```python
from build123d import *

# Parameters (mm, degrees)
SKETCH2_W               = 30
SKETCH2_H               = 18.5
BOSS_EXTRUDE1_DEPTH     = 4.5
BOSS_EXTRUDE2_DEPTH     = 5
SKETCH4_W               = 26.3
SKETCH4_H               = 37.3
BOSS_EXTRUDE3_DEPTH     = 9
SKETCH5_W               = 30
SKETCH5_H               = 40.415903306
SKETCH5_W_2             = 26.3
SKETCH5_H_2             = 37.3
BOSS_EXTRUDE4_DEPTH     = 2
CUT_EXTRUDE1_DEPTH      = 53.877515324
SKETCH7_R               = 2.75
CUT_EXTRUDE2_DEPTH      = 3
SKETCH8_R               = 1.65
CUT_EXTRUDE3_DEPTH      = 51.656012741
SKETCH9_W               = 0.2
SKETCH9_H               = 4
TOLERANCE_CUT1_DEPTH    = 53.877515324
TOLERANCE_CUT2_DEPTH    = 0.2
SKETCH12_W              = 26.022193388
SKETCH12_H              = 26.438096694
BOSS_EXTRUDE6_DEPTH     = 1.5
SKETCH13_W              = 28.011096694
SKETCH13_H              = 28.427
BOSS_EXTRUDE7_DEPTH     = 1.5
SKETCH16_W              = 1.5
SKETCH16_H              = 1.5
SILICONE_CHANNELS_DEPTH = 3
SKETCH19_W              = 19.3
SKETCH19_H              = 15.3
PCB_CAVITY_DEPTH        = 1.7
SKETCH15_R              = 1
PCB_MOUNT_HOLES_DEPTH   = 5
SKETCH20_W              = 5
SKETCH20_H              = 15.3
SOLDER_CAVITY_DEPTH     = 1.2
SKETCH21_R              = 0.5
AUDIO_CHANNEL_DEPTH     = 50.204386256
SKETCH22_R              = 3.5
CUT_EXTRUDE13_DEPTH     = 52.193570171


with BuildPart() as part:
    # Sketch2 → Boss-Extrude1 (new body)
    with BuildSketch(Plane.XY):
        with Locations((13, -1.25)):
            Rectangle(SKETCH2_W, SKETCH2_H)
    extrude(amount=BOSS_EXTRUDE1_DEPTH)

    # Sketch3 → Boss-Extrude2 (add)
    with BuildSketch(Plane.XY.offset(4.5)):
        Polygon((-2, 38.415903306), (28, 38.415903306), (28, -6), (22.890598923, -6), (25.2, -2), (0.7, -2), (3.009401077, -6), (-2, -6), align=None)
    extrude(amount=BOSS_EXTRUDE2_DEPTH)

    # Sketch4 → Boss-Extrude3 (add)
    with BuildSketch(Plane.XY.offset(9.5)):
        Polygon((-2, 38.415903306), (-2, -6), (3.009401077, -6), (0.7, -2), (25.2, -2), (22.890598923, -6), (28, -6), (28, 38.415903306), align=None)
        with Locations((13, 18.5)):
            Rectangle(SKETCH4_W, SKETCH4_H, mode=Mode.SUBTRACT)
    extrude(amount=BOSS_EXTRUDE3_DEPTH)

    # Sketch5 → Boss-Extrude4 (add)
    with BuildSketch(Plane.XY.offset(18.5)):
        with Locations((13, 18.207951653)):
            Rectangle(SKETCH5_W, SKETCH5_H)
        with Locations((13, 18.5)):
            Rectangle(SKETCH5_W_2, SKETCH5_H_2, mode=Mode.SUBTRACT)
    extrude(amount=BOSS_EXTRUDE4_DEPTH)

    # Sketch6 → Cut-Extrude1 (cut, through all)
    with BuildSketch(Plane(origin=(28, 0, 0), x_dir=(0, 0, -1), z_dir=(1, 0, 0))):
        with BuildLine():
            Line((-12.5, 38.415903306), (-29.920257518, 38.415903306))
            Line((-29.920257518, 38.415903306), (-29.920257518, -0.15))
            Line((-29.920257518, -0.15), (-20.5, -0.15))
            ThreePointArc((-20.5, -0.15), (-19.694107493, 6.728151663), (-17.320084205, 13.23372208))
            ThreePointArc((-17.320084205, 13.23372208), (-13.721563712, 23.094799932), (-12.5, 33.520632668))
            Line((-12.5, 33.520632668), (-12.5, 38.415903306))
        make_face()
    extrude(amount=-CUT_EXTRUDE1_DEPTH, mode=Mode.SUBTRACT)

    # Sketch7 → Cut-Extrude2 (cut)
    with BuildSketch(Plane(origin=(0, 0, 0), x_dir=(-1, 0, 0), z_dir=(0, 0, -1))):
        with Locations((-19.5, -6.25)):
            Circle(SKETCH7_R)
        with Locations(Location((-6.5, -6.25, 0), (0, 0, 180))):
            Circle(SKETCH7_R)
    extrude(amount=-CUT_EXTRUDE2_DEPTH, mode=Mode.SUBTRACT)

    # Sketch8 → Cut-Extrude3 (cut, through all)
    with BuildSketch(Plane(origin=(0, 0, 3), x_dir=(-1, 0, 0), z_dir=(0, 0, -1))):
        with Locations((-19.5, -6.25)):
            Circle(SKETCH8_R)
        with Locations((-6.5, -6.25)):
            Circle(SKETCH8_R)
    extrude(amount=-CUT_EXTRUDE3_DEPTH, mode=Mode.SUBTRACT)

    # Sketch9 → tolerance_cut1 (cut, through all)
    with BuildSketch(Plane.ZY.offset(2)):
        with Locations((18.4, -4)):
            Rectangle(SKETCH9_W, SKETCH9_H)
    extrude(amount=-TOLERANCE_CUT1_DEPTH, mode=Mode.SUBTRACT)

    # Sketch10 → tolerance_cut2 (cut)
    with BuildSketch(Plane.XY.offset(4.5)):
        Polygon((28, -6), (22.890598923, -6), (25.2, -2), (0.7, -2), (3.009401077, -6), (-2, -6), (-2, -10.5), (28, -10.5), align=None)
    extrude(amount=-TOLERANCE_CUT2_DEPTH, mode=Mode.SUBTRACT)

    # Sketch12 → Boss-Extrude6 (add)
    with BuildSketch(Plane(origin=(0, 0, 4.5), x_dir=(-1, 0, 0), z_dir=(0, 0, -1))):
        with Locations((-13, 23.207951653)):
            Rectangle(SKETCH12_W, SKETCH12_H)
    extrude(amount=BOSS_EXTRUDE6_DEPTH)

    # Sketch13 → Boss-Extrude7 (add)
    with BuildSketch(Plane(origin=(0, 0, 3), x_dir=(-1, 0, 0), z_dir=(0, 0, -1))):
        with Locations((-13, 23.207951653)):
            Rectangle(SKETCH13_W, SKETCH13_H)
    extrude(amount=BOSS_EXTRUDE7_DEPTH)

    # Sketch16 → silicone_channels (cut)
    with BuildSketch(Plane(origin=(0, 0, 1.5), x_dir=(-1, 0, 0), z_dir=(0, 0, -1))):
        with Locations((-25.261096694, 25.419380652)):
            Rectangle(SKETCH16_W, SKETCH16_H)
        with Locations((-25.261096694, 31.419380652)):
            Rectangle(SKETCH16_W, SKETCH16_H)
        with Locations((-25.261096694, 19.419380652)):
            Rectangle(SKETCH16_W, SKETCH16_H)
        with Locations((-25.261096694, 13.419380652)):
            Rectangle(SKETCH16_W, SKETCH16_H)
        with Locations((-21.014935628, 10.738903306)):
            Rectangle(SKETCH16_W, SKETCH16_H)
        with Locations((-19.514935628, 35.677)):
            Rectangle(SKETCH16_W, SKETCH16_H)
        with Locations((-4.985064372, 10.738903306)):
            Rectangle(SKETCH16_W, SKETCH16_H)
        with Locations((-0.738903306, 13.419380652)):
            Rectangle(SKETCH16_W, SKETCH16_H)
        with Locations((-0.738903306, 19.419380652)):
            Rectangle(SKETCH16_W, SKETCH16_H)
        with Locations((-0.738903306, 25.419380652)):
            Rectangle(SKETCH16_W, SKETCH16_H)
        with Locations((-0.738903306, 31.419380652)):
            Rectangle(SKETCH16_W, SKETCH16_H)
        with Locations((-6.485064372, 35.677)):
            Rectangle(SKETCH16_W, SKETCH16_H)
    extrude(amount=-SILICONE_CHANNELS_DEPTH, mode=Mode.SUBTRACT)

    # Sketch19 → pcb_cavity (cut)
    with BuildSketch(Plane.XY.offset(9.5)):
        with Locations((13, 29.5)):
            Rectangle(SKETCH19_W, SKETCH19_H)
    extrude(amount=-PCB_CAVITY_DEPTH, mode=Mode.SUBTRACT)

    # Sketch15 → pcb_mount_holes (cut)
    with BuildSketch(Plane.XY.offset(7.8)):
        with Locations((13, 34.5)):
            Circle(SKETCH15_R)
        with Locations((13, 24.5)):
            Circle(SKETCH15_R)
    extrude(amount=-PCB_MOUNT_HOLES_DEPTH, mode=Mode.SUBTRACT)

    # Sketch20 → solder_cavity (cut)
    with BuildSketch(Plane.XY.offset(7.8)):
        with Locations((5.85, 29.5)):
            Rectangle(SKETCH20_W, SKETCH20_H)
        with Locations((20.15, 29.5)):
            Rectangle(SKETCH20_W, SKETCH20_H)
    extrude(amount=-SOLDER_CAVITY_DEPTH, mode=Mode.SUBTRACT)

    # Sketch21 → audio_channel (cut, through all)
    with BuildSketch(Plane.XY.offset(7.8)):
        with Locations((13, 29.5)):
            Circle(SKETCH21_R)
    extrude(amount=-AUDIO_CHANNEL_DEPTH, mode=Mode.SUBTRACT)

    # Sketch22 → Cut-Extrude13 (cut, through all)
    with BuildSketch(Plane(origin=(0, 0, 1.5), x_dir=(-1, 0, 0), z_dir=(0, 0, -1))):
        with Locations((-13, 29.5)):
            Circle(SKETCH22_R)
    extrude(amount=-CUT_EXTRUDE13_DEPTH, mode=Mode.SUBTRACT)


solid = part.part
```
Read the model definition and answer for the solid it produces. Units are mm, in the model's axes. A direction names the side the tool comes from. Coordinates: 2 decimals unless noted, no trailing zeros. Write each loop counter-clockwise with the first axis right and the second up, starting at its lowest first coordinate (ties: lowest second). Pieces come first, ordered by that corner, then holes. Notation, with made-up numbers: (64, -9) - (100, -9) arc R20 ccw to (100, 30) - close; hole circle Ø7 at (3, 5.25). An arc over 180 degrees is marked (long way). Answer as a JSON object with one key per item and string values. Group by question number.
1. Consider L1, parallel to Y at x = 13, z = 4.85; L2, parallel to X at y = 25, z = 2; L3, parallel to Y at x = 13, z = 4.15. Determine where each line is inside the solid, lowest interval first. Write a range as [from, to].
2. The mould has two halves that part along Y. Classify faces 1 (the flat face through (25, 26.169, 3)), 2 (the cylindrical face through (27.088, 22.952, 13.756)), 3 (the flat face through (20.265, 11, 3)), 4 (the flat face through (13, -1, 20.5)): +Y half, -Y half, draft (parallel to the pull), parting line (faces both ways), or undercut.
3. A cutting plane is placed at B-B (z = 5). Determine the outline of the cut face in (x, y), plus the area to 3 significant figures.
4. A cutting plane is placed at C-C (x = 19.5). Give the number of separate pieces and of enclosed holes in the cut face, plus the area to 3 significant figures.
5. Which of the six approach directions +Z, -Z, +X, -X, +Y, -Y give full straight-line access (tool end or side, diameter ignored) to faces 5 (the flat face through (0, -4, 18.3)), 6 (the flat face through (-0.011, 22, 4)), 7 (the flat face through (25, 12.669, 3)), 8 (the flat face through (26.15, 14, 14)), 9 (the flat face through (13, 9.989, 4))?
6. Each of these flat-tipped pins is pushed along its axis until it touches: P1, Ø1.6, axis at y = 25, z = 2.5, coming from the +X side; P2, Ø6, axis at x = 4.5, y = 11, coming from the +Z side; P3, Ø0.8, axis at y = 22.5, z = 4, coming from the +X side; P4, Ø12, axis at x = 15.5, z = 17.5, coming from the +Y side. Where does it stop, or does it pass through?
7. A cutting plane is placed at D-D (z = 9). Determine the outline of the cut face in (x, y), plus the area to 3 significant figures.
Worked out:
{
 "1": {"L1": "y = [-2, 23.5], [25.5, 26], [33, 33.5], [35.5, 38.42]", "L2": "x = [-1.01, -0.01], [1.49, 24.51], [26.01, 27.01]", "L3": "y = [-10.5, 8], [9.99, 23.5], [25.5, 26], [33, 33.5], [35.5, 36.43]"},
 "2": {"face 1": "undercut", "face 2": "+Y half", "face 3": "undercut", "face 4": "draft"},
 "3": {"outline": "(-2, -6) - (3.01, -6) - (0.7, -2) - (25.2, -2) - (22.89, -6) - (28, -6) - (28, 38.42) - (-2, 38.42) - close; hole circle Ø7 at (13, 29.5); hole circle Ø2 at (13, 24.5); hole circle Ø2 at (13, 34.5)", "area": "1,200 mm²"},
 "4": {"separate pieces": "3", "enclosed holes": "0", "area": "320 mm²"},
 "5": {"face 5": "+Z, +X, -X, -Y", "face 6": "-X, +Y", "face 7": "-Z", "face 8": "+Z", "face 9": "+X, -X"},
 "6": {"P1": "stops at x = 27.01", "P2": "stops at z = 9.5", "P3": "stops at x = 26.01", "P4": "stops at y = 38.42"},
 "7": {"outline": "(-2, -6) - (3.01, -6) - (0.7, -2) - (25.2, -2) - (22.89, -6) - (28, -6) - (28, 38.42) - (-2, 38.42) - close; hole (3.35, 21.85) - (22.65, 21.85) - (22.65, 37.15) - (3.35, 37.15) - close", "area": "948 mm²"}
}
